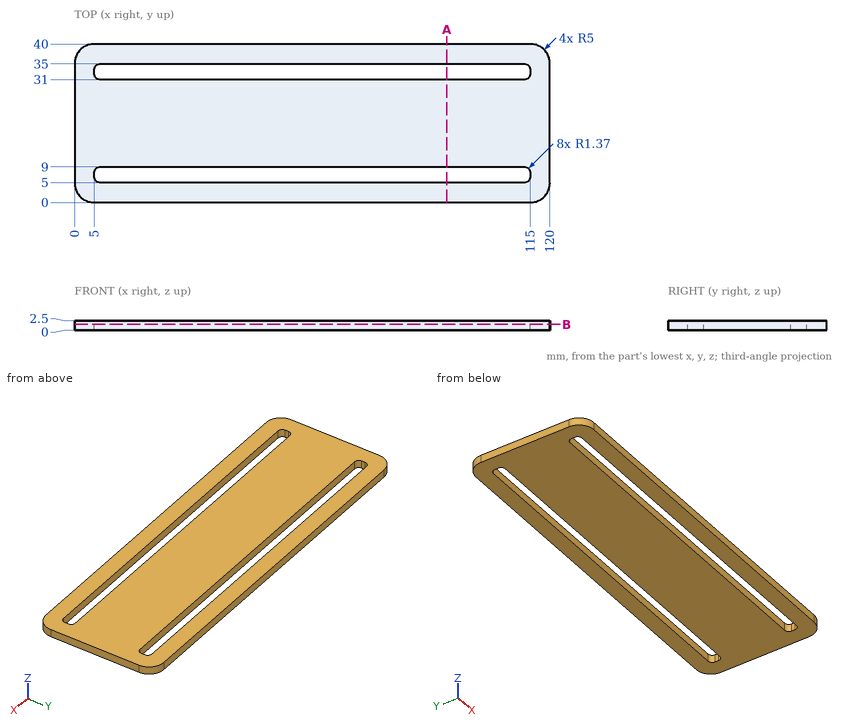
Drawing for the job (mm, zero at the part's lowest x, y, z). Coordinates: 2 decimals unless noted, no trailing zeros. Order: outer loops, then holes, each group sorted by start corner. A loop starts at its lowest first (then second) coordinate and runs counter-clockwise, first axis right, second up.
Item 1: Band-saw the part on B-B on z = 1.5. List the corners of the cut face in (x, y).
Check sheet entries:
outline: (0, 5) arc R5 ccw to (5, 0) - (115, 0) arc R5 ccw to (120, 5) - (120, 35) arc R5 ccw to (115, 40) - (5, 40) arc R5 ccw to (0, 35) - close; hole (5, 6.37) arc R1.37 ccw to (6.37, 5) - (113.63, 5) arc R1.37 ccw to (115, 6.37) - (115, 7.63) arc R1.37 ccw to (113.63, 9) - (6.37, 9) arc R1.37 ccw to (5, 7.63) - close; hole (5, 32.37) arc R1.37 ccw to (6.37, 31) - (113.63, 31) arc R1.37 ccw to (115, 32.37) - (115, 33.63) arc R1.37 ccw to (113.63, 35) - (6.37, 35) arc R1.37 ccw to (5, 33.63) - close
Item 2: Drill centre lines: L1, parallel to Y at x = 7, z = 2.05; L2, parallel to X at y = 35.5, z = 1 (3 decimals); L3, parallel to X at y = 7.5, z = 0.6. Where is each one in solid material? Low to high.
Check sheet entries:
L1: y = 0 to 5, 9 to 31, 35 to 40
L2: x = 0.025 to 119.975
L3: x = 0 to 5, 115 to 120
Item 3: Band-saw the part on A-A on x = 94. List the corners of the cut face in (y, z).
Check sheet entries:
outline: (0, 0) - (5, 0) - (5, 2.5) - (0, 2.5) - close; (9, 0) - (31, 0) - (31, 2.5) - (9, 2.5) - close; (35, 0) - (40, 0) - (40, 2.5) - (35, 2.5) - close
